```python
from build123d import *

# Parameters (mm, degrees)
SKETCH_2_W           = 27.5
SKETCH_2_H           = 3
EXTRUDE_1_DEPTH      = 46.8
SKETCH_3_R           = 1
CUT_EXTRUDE_1_DEPTH  = 46.8
EXTRUDE_2_DEPTH      = 25
EXTRUDE_2_DEPTH_BACK = 25
SKETCH_4_W           = 3
SKETCH_4_H           = 20
SKETCH_5_R           = 1.5
CUT_EXTRUDE_2_DEPTH  = 25


with BuildPart() as part:
    # 草图2 → 凸台-拉伸1 (new body)
    with BuildSketch(Plane(origin=(0, 0, 0), x_dir=(1, 0, 0), z_dir=(0, 1, 0))):
        Rectangle(SKETCH_2_W, SKETCH_2_H)
    extrude(amount=EXTRUDE_1_DEPTH)

    # 草图3 → 切除-拉伸1 (cut)
    with BuildSketch(Plane(origin=(0, 0, -1.5), x_dir=(-1, 0, 0), z_dir=(0, 0, -1))):
        with Locations((-12.3, 44.893116562)):
            Circle(SKETCH_3_R)
        with Locations((-12.3, 2.2)):
            Circle(SKETCH_3_R)
        with Locations((12.3, 2.2)):
            Circle(SKETCH_3_R)
        with Locations((12.3, 44.893116562)):
            Circle(SKETCH_3_R)
    extrude(amount=-CUT_EXTRUDE_1_DEPTH, mode=Mode.SUBTRACT)

    # 草图4 → 凸台-拉伸2 (add, two sides: drawn at the far end of the back side and taken through both)
    with BuildSketch(Plane(origin=(0, 0, 0), x_dir=(0, 0, -1), z_dir=(1, 0, 0)).offset(-EXTRUDE_2_DEPTH_BACK)):
        with Locations((0, 23.4)):
            Rectangle(SKETCH_4_W, SKETCH_4_H)
    extrude(amount=EXTRUDE_2_DEPTH + EXTRUDE_2_DEPTH_BACK)

    # 草图5 → 切除-拉伸2 (cut)
    with BuildSketch(Plane(origin=(0, 0, -1.5), x_dir=(-1, 0, 0), z_dir=(0, 0, -1))):
        with Locations((-22, 23.4)):
            Circle(SKETCH_5_R)
        with Locations((22, 23.4)):
            Circle(SKETCH_5_R)
    extrude(amount=-CUT_EXTRUDE_2_DEPTH, mode=Mode.SUBTRACT)


solid = part.part
```
Can you work these out from the model? Positions are in its coordinate system, mm. A direction names the side the tool comes from. Round coordinates to 2 decimals unless told otherwise and drop trailing zeros. Loops run counter-clockwise (first coordinate to the right, second up) from the corner with the lowest first, then second, coordinate; pieces in that order, holes last. Notation, with made-up numbers: M 86.5,62.5 L 126.5,62.5 A30 ccw 126.5,84.5 Z; hole C 14,7.25 d11. An arc over 180 degrees is marked long. Answer in a Markdown table with one row per item.
1. If we section it at A-A, the plane x = 12.3: Please give me the cut outline in (y, z).
Established:
| item | result |
|---|---|
| outline | M 0,-1.5 L 1.2,-1.5 L 1.2,1.5 L 0,1.5 Z; M 3.2,-1.5 L 43.89,-1.5 L 43.89,1.5 L 3.2,1.5 Z; M 45.89,-1.5 L 46.8,-1.5 L 46.8,1.5 L 45.89,1.5 Z |
2. If we section it at B-B, the plane y = 23.4: Please give me the cut outline in (x, z), plus the area to 3 significant figures.
Established:
| item | result |
|---|---|
| outline | M -25,-1.5 L -23.5,-1.5 L -23.5,1.5 L -25,1.5 Z; M -20.5,-1.5 L 20.5,-1.5 L 20.5,1.5 L -20.5,1.5 Z; M 23.5,-1.5 L 25,-1.5 L 25,1.5 L 23.5,1.5 Z |
| area | 132 mm² |
3. If we section it at C-C, the plane x = -22: Please give me the cut outline in (y, z), plus the area to 3 significant figures.
Established:
| item | result |
|---|---|
| outline | M 13.4,-1.5 L 21.9,-1.5 L 21.9,1.5 L 13.4,1.5 Z; M 24.9,-1.5 L 33.4,-1.5 L 33.4,1.5 L 24.9,1.5 Z |
| area | 51.0 mm² |
4. If we section it at D-D, the plane z = 0.4: Please give me the cut outline in (x, y).
Established:
| item | result |
|---|---|
| outline | M -25,13.4 L -13.75,13.4 L -13.75,0 L 13.75,0 L 13.75,13.4 L 25,13.4 L 25,33.4 L 13.75,33.4 L 13.75,46.8 L -13.75,46.8 L -13.75,33.4 L -25,33.4 Z; hole C -22,23.4 d3; hole C -12.3,2.2 d2; hole C -12.3,44.89 d2; hole C 12.3,2.2 d2; hole C 12.3,44.89 d2; hole C 22,23.4 d3 |
5. Thinking about a two-plate mould opening in X: for faces 6 (the face through (0, 23, -1.5)), 7 (the face through (-12.761, 44.006, -0.021)), 8 (the face through (-25, 24, 0)), 9 (the face through (13.75, 7, 0)), which applies, pulls with the +X half, pulls with the -X half, needs draft (parallel to the pull), parting line crosses it, or undercut?
Established:
| item | result |
|---|---|
| face 6 | needs draft |
| face 7 | undercut |
| face 8 | pulls with the -X half |
| face 9 | pulls with the +X half |
6. On a 3-axis mill with a long thin cutter (end or side, diameter ignored), from which of +Z, -Z, +X, -X, +Y, -Y can I reach the whole of each face in a straight line? I mean faces 1 (the face through (-13.75, 7, 0)), 2 (the face through (19, 33.4, 0)), 3 (the face through (-13.75, 40, 0)), 4 (the face through (-20.5, 23.47, -0.02)), 5 (the face through (19, 13.4, 0)). Say none if no direction works.
Established:
| item | result |
|---|---|
| face 1 | +Z, -Z, -X, -Y |
| face 2 | +Z, -Z, +X, +Y |
| face 3 | +Z, -Z, -X, +Y |
| face 4 | +Z, -Z |
| face 5 | +Z, -Z, +X, -Y |
7. Please list where these lines run through material, in increasing order: line 1 (Y direction, x = 12.3, z = -0.15); line 2 (Y direction, x = 22, z = 0.1); line 3 (X direction, y = 23, z = -0.7). Write a range as from..to.
Established:
| item | result |
|---|---|
| line 1 | 0..1.2, 3.2..43.89, 45.89..46.8 |
| line 2 | 13.4..21.9, 24.9..33.4 |
| line 3 | -25..-23.45, -20.55..20.55, 23.45..25 |
8. I'm going to push a flat-ended pin straight in: pin 1 Ø0.9 at (y, z) = (42.5, 0.5) entering from +X. Where does the tip first touch, or does it pass through?
Established:
| item | result |
|---|---|
| pin 1 | x = 13.75 |
